Geometry check sheet. Reference: the model listing, model coordinates, mm. Face numbers are marked on the shaded views. Coordinates: 2 decimals unless noted, no trailing zeros. Order: outer loops, then holes, each group sorted by start corner. A loop starts at its lowest first (then second) coordinate and runs counter-clockwise, first axis right, second up. Notation, with made-up numbers: (85, 44.5) - (113, 44.5) arc R13 cw to (113, 55.5) - close; hole circle Ø5 at (3.5, 46.5). An arc over 180 degrees is marked (long way). Return JSON: item names as keys, results as strings. Group by question number.
Item 1: Draft check along Z on the marked faces 1 and 2. Enter one of: pulls with the +Z half, pulls with the -Z half, needs draft (parallel to the pull), parting line crosses it, or undercut.
Item 2: Section check C-C on x = 7. Enter the section's corners in (y, z).
Item 3: Scan lines: probe 1 along X at (y, z) = (2.5, 28); probe 2 along Z at (x, y) = (16, 2.7); probe 3 along X at (y, z) = (2.5, 21). Record each from-to range of solid material in increasing order.
Item 4: Section check A-A on x = 25. Enter the section's corners in (y, z).
Item 5: Section check D-D on z = 12. Enter the section's corners in (x, y), then the cut area to 3 significant figures.
Item 6: Gauge pin test, flat end, axial feed: pin 1 (6 mm diameter, centred on x = 7, z = -9.5, fed in from +Y). Record the tip position at first contact, or that the pin passes through.
Item 7: Section check B-B on y = 3.35. Enter the section's corners in (x, z), then the cut area to 3 significant figures.
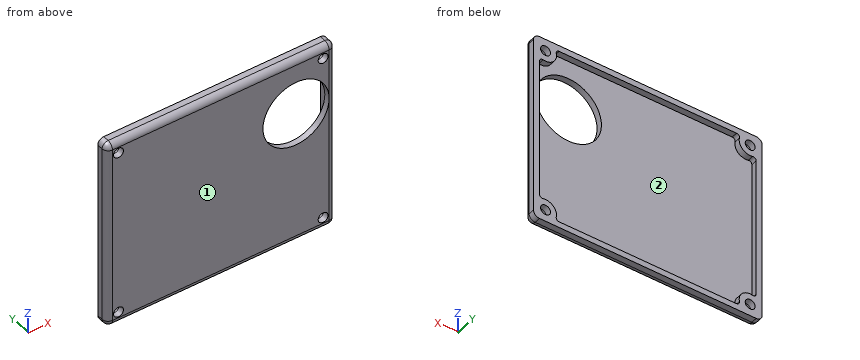
from build123d import *

# Parameters (mm, degrees)
SCHIZZO1_W                   = 76
SCHIZZO1_H                   = 64
ESTRUSIONE_ESTRUSIONE1_DEPTH = 4
SCHIZZO2_W                   = 72
SCHIZZO2_H                   = 60
TAGLIO_ESTRUSIONE1_DEPTH     = 2
SCHIZZO3_R                   = 3.65
SCHIZZO3_R_2                 = 1.65
ESTRUSIONE_ESTRUSIONE2_DEPTH = 2
SCHIZZO3_11_R                = 1.65
TAGLIO_ESTRUSIONE4_DEPTH     = 50.719211579
SCHIZZO5_R                   = 11
TAGLIO_ESTRUSIONE5_DEPTH     = 2
RACCORDO1_R                  = 1
RACCORDO2_R                  = 2


with BuildPart() as part:
    # Schizzo1 → Estrusione-Estrusione1 (new body)
    with BuildSketch(Plane(origin=(0, 0, 0), x_dir=(1, 0, 0), z_dir=(0, 1, 0))):
        Rectangle(SCHIZZO1_W, SCHIZZO1_H)
    extrude(amount=ESTRUSIONE_ESTRUSIONE1_DEPTH)

    # Schizzo2 → Taglio-Estrusione1 (cut)
    with BuildSketch(Plane(origin=(0, 4, 0), x_dir=(1, 0, 0), z_dir=(0, 1, 0))):
        Rectangle(SCHIZZO2_W, SCHIZZO2_H)
    extrude(amount=-TAGLIO_ESTRUSIONE1_DEPTH, mode=Mode.SUBTRACT)

    # Schizzo3 → Estrusione-Estrusione2 (add)
    # profile 1 of 4: a face of its own
    with BuildSketch(Plane(origin=(0, 2, 0), x_dir=(1, 0, 0), z_dir=(0, 1, 0))):
        with Locations((34, 28)):
            Circle(SCHIZZO3_R)
        with Locations(Location((34, 28, 0), (0, 0, 270))):
            Circle(SCHIZZO3_R_2, mode=Mode.SUBTRACT)
    # profile 2 of 4: a face of its own
    with BuildSketch(Plane(origin=(0, 2, 0), x_dir=(1, 0, 0), z_dir=(0, 1, 0))):
        with Locations((-34, 28)):
            Circle(SCHIZZO3_R)
        with Locations(Location((-34, 28, 0), (0, 0, 270))):
            Circle(SCHIZZO3_R_2, mode=Mode.SUBTRACT)
    # profile 3 of 4: a face of its own
    with BuildSketch(Plane(origin=(0, 2, 0), x_dir=(1, 0, 0), z_dir=(0, 1, 0))):
        with Locations((34, -28)):
            Circle(SCHIZZO3_R)
        with Locations(Location((34, -28, 0), (0, 0, 270))):
            Circle(SCHIZZO3_R_2, mode=Mode.SUBTRACT)
    # profile 4 of 4: a face of its own
    with BuildSketch(Plane(origin=(0, 2, 0), x_dir=(1, 0, 0), z_dir=(0, 1, 0))):
        with Locations((-34, -28)):
            Circle(SCHIZZO3_R)
        with Locations(Location((-34, -28, 0), (0, 0, 270))):
            Circle(SCHIZZO3_R_2, mode=Mode.SUBTRACT)
    extrude(amount=ESTRUSIONE_ESTRUSIONE2_DEPTH)

    # Schizzo3<11> → Taglio-Estrusione4 (cut, through all)
    with BuildSketch(Plane(origin=(0, 2, 0), x_dir=(1, 0, 0), z_dir=(0, 1, 0))):
        with Locations(Location((-34, 28, 0), (0, 0, 270))):
            Circle(SCHIZZO3_11_R)
        with Locations(Location((-34, -28, 0), (0, 0, 270))):
            Circle(SCHIZZO3_11_R)
        with Locations(Location((34, -28, 0), (0, 0, 270))):
            Circle(SCHIZZO3_11_R)
        with Locations(Location((34, 28, 0), (0, 0, 270))):
            Circle(SCHIZZO3_11_R)
    extrude(amount=-TAGLIO_ESTRUSIONE4_DEPTH, mode=Mode.SUBTRACT)

    # Schizzo5 → Taglio-Estrusione5 (cut)
    with BuildSketch(Plane.XZ):
        with Locations(Location((25, 13, 0), (0, 0, 270))):
            Circle(SCHIZZO5_R)
    extrude(amount=-TAGLIO_ESTRUSIONE5_DEPTH, mode=Mode.SUBTRACT)

    # Raccordo1
    raccordo1_edges = [part.edges().sort_by_distance(p)[0] for p in [
        (30.946723072, 3, -30),
        (36, 3, -24.946723072),
        (-36, 3, -24.946723072),
        (-30.946723072, 3, -30),
        (-30.946723072, 3, 30),
        (-36, 3, 24.946723072),
        (36, 3, 24.946723072),
        (30.946723072, 3, 30),
    ]]
    fillet(raccordo1_edges, radius=RACCORDO1_R)

    # Raccordo2
    raccordo2_edges = [part.edges().sort_by_distance(p)[0] for p in [
        (0, 0, 32),
        (-38, 0, 0),
        (0, 0, -32),
        (38, 0, 0),
        (38, 2, 32),
        (-38, 2, 32),
        (-38, 2, -32),
        (38, 2, -32),
    ]]
    fillet(raccordo2_edges, radius=RACCORDO2_R - 0.0001)  # a hair under: the kernel refuses the full size


solid = part.part
Computed:
{
 "1": {"face 1": "needs draft", "face 2": "undercut"},
 "2": {"outline": "(0, -30) arc R2 ccw to (2, -32) - (4, -32) - (4, -30) - (2, -30) - (2, 30) - (4, 30) - (4, 32) - (2, 32) arc R2 ccw to (0, 30) - close"},
 "3": {"probe 1": "x = -38 to -35.65, -32.35 to -30.35, 30.35 to 32.35, 35.65 to 38", "probe 2": "z = -32 to -30, 30 to 32", "probe 3": "x = -38 to -36, 36 to 38"},
 "4": {"outline": "(0, -30) arc R2 ccw to (2, -32) - (4, -32) - (4, -30) - (2, -30) - (2, 2) - (0, 2) - close; (0, 24) - (2, 24) - (2, 30) - (4, 30) - (4, 32) - (2, 32) arc R2 ccw to (0, 30) - close"},
 "5": {"outline": "(-38, 2) arc R2 ccw to (-36, 0) - (14.05, 0) - (14.05, 2) - (-36, 2) - (-36, 4) - (-38, 4) - close; (35.95, 0) - (36, 0) arc R2 ccw to (38, 2) - (38, 4) - (36, 4) - (36, 2) - (35.95, 2) - close", "area": "114 mm²"},
 "6": {"pin 1": "stops at y = 2"},
 "7": {"outline": "(-38, -30) arc R2 ccw to (-36, -32) - (36, -32) arc R2 ccw to (38, -30) - (38, 30) arc R2 ccw to (36, 32) - (-36, 32) arc R2 ccw to (-38, 30) - close; hole (-36, -23.46) arc R1 ccw to (-34.78, -24.44) arc R3.65 cw to (-30.44, -28.78) arc R1 ccw to (-29.46, -30) - (29.46, -30) arc R1 ccw to (30.44, -28.78) arc R3.65 cw to (34.78, -24.44) arc R1 ccw to (36, -23.46) - (36, 23.46) arc R1 ccw to (34.78, 24.44) arc R3.65 cw to (30.44, 28.78) arc R1 ccw to (29.46, 30) - (-29.46, 30) arc R1 ccw to (-30.44, 28.78) arc R3.65 cw to (-34.78, 24.44) arc R1 ccw to (-36, 23.46) - close; hole circle Ø3.3 at (-34, -28); hole circle Ø3.3 at (-34, 28); hole circle Ø3.3 at (34, -28); hole circle Ø3.3 at (34, 28)", "area": "623 mm²"}
}
